Geometry: final body of the model. Coordinates: model frame, mm. A direction names the side the tool comes from. Give positions to 0.01 mm unless a question says otherwise; leave off trailing zeros. Loops run counter-clockwise (first coordinate to the right, second up) from the corner with the lowest first, then second, coordinate; pieces in that order, holes last.
1. Section A-A, the plane y = 33. Output: boundary loops of the cut face in (x, z).
2. Material intervals for line 1 along Z through (x, y) = (-43, 60.5); line 2 along Z through (x, y) = (-23, 38); line 3 along Y through (x, z) = (-51.5, 6.5), sorted ascending.
3. Draft query along X for faces 5 (the face through (-20.35, 45.51, 14.03)), 6 (the face through (-25.944, 64.947, 8.874)), 7 (the face through (-34, 49, 16)). Return one class per face: +X half, -X half, draft (parallel to the pull), parting line (faces both ways), or undercut.
4. First-contact query: P1, Ø2.5, axis at x = -19.59, y = 43.66, coming from the +Z side; P2, Ø11.5, axis at x = -38.5, y = 47.5, coming from the -Z side; P3, Ø2, axis at x = -51.5, z = 1, coming from the +Y side; P4, Ø2, axis at y = 57.5, z = -2.5, coming from the +X side. Flat tips, straight axial feed; report the tip coordinate or a pass-through.
5. Section B-B, the plane z = -6. Output: boundary loops of the cut face in (x, y), then the cut area to 3 significant figures.
6. Access query for faces 1 (the face through (-20.26, 54.177, 14.028)), 2 (the face through (-43.98, 37.57, 14.03)), 3 (the face through (-34, 48, 12)), 4 (the face through (-28.445, 63.289, 8.013)). Directions: +Z, -Z, +X, -X, +Y, -Y. A direction counts if a zero-diameter tool reaches every point of the face in a straight line with its end or side. Return the directions, or none.
7. Section C-C, the plane y = 40. Output: boundary loops of the cut face in (x, z).
from build123d import *

# Parameters (mm, degrees)
SKETCH084_R             = 5
PAD062_DEPTH            = 3
SKETCH085_W             = 26
SKETCH085_H             = 4
PAD063_DEPTH            = 30
SKETCH086_R             = 2
POCKET029_DEPTH         = 31.001
SKETCH087_R             = 1
POCKET030_DEPTH         = 137.42322
POLARPATTERN012_COUNT   = 4
PAD104_DEPTH            = 3
PAD105_DEPTH            = 3
BODY038_PLACEMENT_ANGLE = 35


with BuildPart() as part:
    # Sketch084 → Pad062 (new body)
    with BuildSketch(Plane.XZ):
        with BuildLine():
            Line((-13, 18), (13, 18))
            Line((13, 18), (13, 0))
            ThreePointArc((-13, 0), (0, -13), (13, 0))
            Line((-13, 18), (-13, 0))
        make_face()
        Circle(SKETCH084_R, mode=Mode.SUBTRACT)
    extrude(amount=PAD062_DEPTH)

    # Sketch085 (on Face7 of Pad062) → Pad063 (join)
    with BuildSketch(Plane.XZ.offset(3)):
        with Locations((0, 16)):
            Rectangle(SKETCH085_W, SKETCH085_H)
    extrude(amount=PAD063_DEPTH)

    # Sketch086 (on Face5 of Pad063) → Pocket029 (cut, through all)
    with BuildSketch(Plane(origin=(0, 0, 18), x_dir=(-1, 0, 0), z_dir=(0, 0, 1))):
        with Locations((-9, 7)):
            Circle(SKETCH086_R)
        with Locations((9, 7)):
            Circle(SKETCH086_R)
        with Locations((-9, 29)):
            Circle(SKETCH086_R)
        with Locations((9, 29)):
            Circle(SKETCH086_R)
    extrude(amount=-POCKET029_DEPTH, mode=Mode.SUBTRACT)

    # Sketch087 (on Face4 of Pocket029) → Pocket030 (cut, through all)
    with BuildSketch(Plane(origin=(0, 0, 0), x_dir=(1, 0, 0), z_dir=(0, 1, 0))):
        with Locations((0, 9.5)):
            Circle(SKETCH087_R)
    pocket030 = extrude(amount=-POCKET030_DEPTH, mode=Mode.SUBTRACT)

    # PolarPattern012: Pocket030 ×4 about axis
    polarpattern012_axis = Axis((0, 0, 0), (0, 1, 0))
    for i in range(1, POLARPATTERN012_COUNT):
        add(pocket030.rotate(polarpattern012_axis, i * 360 / POLARPATTERN012_COUNT), mode=Mode.SUBTRACT)

    # Sketch263 (on Face7 of PolarPattern012) → Pad104 (join)
    with BuildSketch(Plane(origin=(-13, 0, 0), x_dir=(0, 0, -1), z_dir=(-1, 0, 0))):
        Polygon((0, 0), (-18, 0), (-18, 20), (-14, 20), (0, 3), align=None)
    extrude(amount=PAD104_DEPTH)

    # Sketch264 (on Face10 of Pad104) → Pad105 (join)
    with BuildSketch(Plane(origin=(13, 0, 0), x_dir=(0, 0, 1), z_dir=(1, 0, 0))):
        Polygon((0, 0), (18, 0), (18, 20), (14, 20), (0, 3), align=None)
    extrude(amount=PAD105_DEPTH)


with BuildPart() as part_1:
    # Body038 placement: moved
    add(part.part.moved(Location((-43.591809, 62.255555, -2))).rotate(Axis((-43.591809, 62.255555, -2), (0, 0, 1)), BODY038_PLACEMENT_ANGLE))


solid = part_1.part
Answers below:
1. outline: (-38.98, 12) - (-36.3, 12) - (-36.3, 16) - (-38.98, 16) - close; (-32.36, 12) - (-27.84, 12) - (-27.84, 16) - (-32.36, 16) - close
2. line 1: z = -14.99 to -12.35, -10.65 to -6.97, 2.97 to 6.65, 8.35 to 16
2. line 2: z = 12 to 16
2. line 3: y = 45.65 to 50.88, 53.06 to 56.72
3. face 5: undercut
3. face 6: +X half
3. face 7: draft
4. P1: passes through
4. P2: stops at z = 12
4. P3: stops at y = 57.42
4. P4: stops at x = -45.81
5. outline: (-53.72, 55.16) - (-52, 52.7) - (-44.33, 58.08) - (-46.05, 60.53) - close; (-41.13, 63.98) - (-39.41, 61.52) - (-31.74, 66.89) - (-33.46, 69.35) - close
5. area: 56.2 mm2
6. face 1: +Z, -Z, +X
6. face 2: +Z, -Z, -Y
6. face 3: -Z
6. face 4: -Z, -Y
7. outline: (-47.54, 8.68) - (-43.88, 10.41) - (-43.88, 12) - (-17.84, 12) - (-17.84, 16) - (-47.54, 16) - close
